Design review of the part built by this model. Coordinates are the model's own, in mm. A direction names the side the tool comes from. Coordinates: 2 decimals unless noted, no trailing zeros. Loops run counter-clockwise (first coordinate to the right, second up) from the corner with the lowest first, then second, coordinate; pieces in that order, holes last.
Q1. For P1, Ø1.8, axis at y = 70.5, z = 743.5, coming from the +X side; P2, Ø5, axis at y = 229.5, z = 343, coming from the +X side; P3, Ø1.8, axis at x = 0.5, z = 725, coming from the +Y side, all flat-tipped, find the tip position at first contact; note any pin that passes through.
Q2. Add section D-D on x = 281.5. Give the boundary of the cut face in (y, z).
Q3. Machinability: for faces 5 (the face through (18, 513, 1.6)), 6 (the face through (91.235, 710.688, 0.789)), which of the approach directions +Z, -Z, +X, -X, +Y, -Y give a long, thin tool a straight path to every point of the face, cutting with its end or side? Answer none if there is none.
Q4. Add section C-C on y = 152.5. Give the boundary of the cut face in (x, z).
Q5. Draft analysis for pull direction Z (two halves, no side actions). For faces 1 (the face through (18, 518, 0)), 2 (the face through (76, 726, 572)), 3 (the face through (16, 518, 1160)), 4 (the face through (1.6, 291, 588)), state which applies: released by +Z, released by -Z, zero draft, split by the parting line, or undercut.
Q6. Add section A-A on z = 311. Give the boundary of the cut face in (x, y), and give its area (3 significant figures).
Q7. Add section B-B on y = 506.5. Give the boundary of the cut face in (x, z).
Q8. Wall thickness on probe 1 along Y at (x, z) = (192, 561.5); probe 2 along X at (y, z) = (236, 797); probe 3 along Y at (x, z) = (113.5, 1086): over which ranges is each line inside the solid? List them lowest first.
Autodesk Inventor part; units mm, degrees
ref_plane "YZ Plane" through (0, 0, 0) normal (1, 0, 0) x (0, 1, 0)
ref_plane "XZ Plane" through (0, 0, 0) normal (0, 1, 0) x (-1, 0, 0)
ref_plane "XY Plane" through (0, 0, 0) normal (0, 0, 1) x (1, 0, 0)
sketch "Sketch1" plane through (0, 0, 0) normal (0, 0, 1) x (1, 0, 0)
  line L0 (150, 800) -> (304, 800)
  line L1 (150, 800) -> (0, 650)
  line L2 (150, 800) -> (1016.5277, 800) construction
  line L3 (0, 650) -> (0, 70)
  line L4 (1.6, 70) -> (1.6, 649.3373)
  line L5 (1.6, 649.3373) -> (150.6627, 798.4)
  line L6 (150.6627, 798.4) -> (304, 798.4)
  line L7 (304, 800) -> (304, 798.4)
  line L8 (0, 70) -> (1.6, 70)
  point P0 (0, 0)
  dimension "d0" = 154
  dimension "d1" = 800
  dimension "d2" = 135
  dimension "d8" = 150
  dimension "d9" = 580
  dimension "d10" = 70
  dimension "d19" = 1.6
extrude "Extrusion1" add sketch "Sketch1" along normal blind 1160
sketch "Sketch2" plane through (0, 70, 0) normal (-1, 0, 0) x (0, 0, 1)
  line L0 (80, 530) -> (1080, 530)
  line L1 (1080, 530) -> (1080, 230)
  line L2 (1080, 230) -> (80, 230)
  line L3 (80, 230) -> (80, 530)
  line L4 (0, 0) -> (0, 580)
  line L5 (0, 580) -> (1160, 580)
  line L6 (0, 0) -> (1160, 0)
  point P0 (0, -70)
  point P1 (580, 230)
  point P2 (580, 0)
  dimension "d13" = 1000
  dimension "d14" = 300
  dimension "d16" = 50
extrude "Extrusion2" cut sketch "Sketch2" against normal through all
sketch "Sketch3" plane through (0, 0, 1160) normal (0, 0, 1) x (1, 0, 0)
  line L0 (150.6627, 798.4) -> (304, 798.4)
  line L1 (1.6, 649.3373) -> (150.6627, 798.4)
  line L2 (1.6, 70) -> (1.6, 649.3373)
  line L3 (304, 778.4) -> (158.947, 778.4)
  line L4 (158.947, 778.4) -> (21.6, 641.053)
  line L5 (21.6, 641.053) -> (21.6, 70)
  line L6 (304, 778.4) -> (304, 798.4)
  line L7 (304, 800) -> (150, 800)
  line L8 (21.6, 70) -> (1.6, 70)
  point P0 (0, 0)
  dimension "d20" = 20
extrude "Extrusion3" add sketch "Sketch3" against normal blind 1.6
sketch "Sketch4" plane through (0, 0, 0) normal (0, 0, -1) x (-1, 0, 0)
  line L0 (-304, 798.4) -> (-150.6627, 798.4)
  line L1 (-304, 798.4) -> (-304, 778.4)
  line L2 (-304, 778.4) -> (-158.947, 778.4)
  line L3 (-158.947, 778.4) -> (-21.6, 641.053)
  line L4 (-21.6, 641.053) -> (-21.6, 70)
  line L5 (-21.6, 70) -> (-1.6, 70)
  line L6 (-1.6, 649.3373) -> (-1.6, 70)
  line L7 (-150.6627, 798.4) -> (-1.6, 649.3373)
  point P0 (0, 0)
extrude "Extrusion4" add sketch "Sketch4" against normal blind 1.6
sketch "Sketch5" plane through (304, 800, 1160) normal (1, 0, 0) x (0, 0, -1)
  line L0 (1158.4, -1.6) -> (1.6, -1.6)
  line L1 (1158.4, -21.6) -> (1158.4, -1.6)
  line L2 (1.6, -1.6) -> (1.6, -21.6)
  line L3 (1.6, -21.6) -> (1.6, -158.947)
  line L4 (1.6, -21.6) -> (1158.4, -21.6)
  point P0 (1160, -800)
extrude "Extrusion5" add sketch "Sketch5" against normal blind 1.6
sketch "Sketch6" plane through (0, 70, 0) normal (0, -1, 0) x (1, 0, 0)
  line L0 (1.6, 1.6) -> (21.6, 1.6)
  line L1 (1.6, 1.6) -> (1.6, 1158.4)
  line L2 (21.6, 1158.4) -> (1.6, 1158.4)
  line L3 (158.947, 1158.4) -> (21.6, 1158.4)
  line L4 (21.6, 1.6) -> (21.6, 1158.4)
  point P0 (0, 0)
extrude "Extrusion6" add sketch "Sketch6" against normal blind 1.6
sketch "Sketch7" plane through (304, 800, 1160) normal (1, 0, 0) x (0, 0, -1)
  line L0 (1.6, -1.6) -> (1.6, -21.6)
  line L1 (1.6, -1.6) -> (3.2, -1.6)
  line L2 (3.2, -1.6) -> (3.2, -21.6)
  line L3 (3.2, -21.6) -> (1.6, -21.6)
  line L4 (1.6, -21.6) -> (1.6, -1.6)
  line L5 (1158.4, -21.6) -> (1158.4, -1.6)
  line L6 (1158.4, -1.6) -> (1156.8, -1.6)
  line L7 (1156.8, -1.6) -> (1156.8, -21.6)
  line L8 (1156.8, -21.6) -> (1158.4, -21.6)
  line L9 (1158.4, -21.6) -> (1158.4, -1.6)
  point P0 (1160, -800)
  dimension "d32" = 1.6
  dimension "d33" = 20
  dimension "d34" = 1.6
  dimension "d35" = 20
extrude "Extrusion7" cut sketch "Sketch7" against normal blind 1.6
sketch "Sketch8" plane through (0, 70, 0) normal (0, -1, 0) x (1, 0, 0)
  line L0 (1.6, 1158.4) -> (1.6, 1.6)
  line L1 (1.6, 1.6) -> (21.6, 1.6)
  line L2 (21.6, 1.6) -> (21.6, 3.2)
  line L3 (21.6, 3.2) -> (1.6, 3.2)
  line L4 (1.6, 3.2) -> (1.6, 1.6)
  line L5 (1.6, 1158.4) -> (21.6, 1158.4)
  line L6 (21.6, 1158.4) -> (21.6, 1156.8)
  line L7 (21.6, 1156.8) -> (1.6, 1156.8)
  line L8 (1.6, 1156.8) -> (1.6, 1158.4)
  point P0 (0, 0)
  dimension "d38" = 20
  dimension "d39" = 1.6
  dimension "d40" = 20
  dimension "d41" = 1.6
extrude "Extrusion8" cut sketch "Sketch8" against normal blind 1.6
properties part number "Front Panel" material "Steel"
Entries:
1. P1: stops at x = 21.6
1. P2: stops at x = 1.6
1. P3: stops at y = 651.4
2. outline: (778.4, 0) - (800, 0) - (800, 1160) - (778.4, 1160) - (778.4, 1158.4) - (798.4, 1158.4) - (798.4, 1.6) - (778.4, 1.6) - close
3. face 5: +X, -Y
3. face 6: +Z, -Z, +X, -Y
4. outline: (0, 0) - (21.6, 0) - (21.6, 1.6) - (1.6, 1.6) - (1.6, 1158.4) - (21.6, 1158.4) - (21.6, 1160) - (0, 1160) - close
5. face 1: released by -Z
5. face 2: zero draft
5. face 3: released by +Z
5. face 4: undercut
6. outline: (0, 70) - (21.6, 70) - (21.6, 71.6) - (1.6, 71.6) - (1.6, 300) - (0, 300) - close; (0, 600) - (1.6, 600) - (1.6, 649.34) - (150.66, 798.4) - (302.4, 798.4) - (302.4, 778.4) - (304, 778.4) - (304, 800) - (150, 800) - (0, 650) - close
6. area: 1,100 mm2
7. outline: (0, 0) - (21.6, 0) - (21.6, 1.6) - (1.6, 1.6) - (1.6, 80) - (0, 80) - close; (0, 1080) - (1.6, 1080) - (1.6, 1158.4) - (21.6, 1158.4) - (21.6, 1160) - (0, 1160) - close
8. probe 1: y = 798.4 to 800
8. probe 2: x = 0 to 1.6
8. probe 3: y = 761.24 to 763.5
